```python
from build123d import *

# Parameters (mm, degrees)
F0_W      = 48
F0_H      = 165
F1_DEPTH  = 3
F2_W      = 5.386259
F2_H      = 60
F1_FACE_W = 48
F1_FACE_H = 165
F3_DEPTH  = 3
F4_W      = 15
F4_H      = 17
F5_DEPTH  = 3
F6_R      = 7
F8_DEPTH  = 61.790481
F10_D     = 3
F15_D     = 3
F17_D     = 3
F19_D     = 3
F21_D     = 3


with BuildPart() as f1:
    # F0 (on Top) → F1 (new body)
    with BuildSketch(Plane.XY):
        with Locations((24, 82.5)):
            Rectangle(F0_W, F0_H)
    extrude(amount=F1_DEPTH)

    # F2 (on face) + F1_face (on face) → F3 (join)
    with BuildSketch(Plane.XY.offset(3)):
        with Locations((50.693129, 30)):
            Rectangle(F2_W, F2_H)
    with BuildSketch(Plane(origin=(24, 82.5, 3), x_dir=(1, 0, 0), z_dir=(0, 0, 1))):
        Rectangle(F1_FACE_W, F1_FACE_H)
    extrude(amount=-F3_DEPTH)

    # F4 (on face) → F5 (join)
    with BuildSketch(Plane.XY.offset(3)):
        with Locations((7.5, 173.5)):
            Rectangle(F4_W, F4_H)
    extrude(amount=-F5_DEPTH)

    # F6
    f6_edges = [f1.edges().sort_by_distance(p)[0] for p in [
        (15, 182, 1.5),
    ]]
    fillet(f6_edges, radius=F6_R)

    # F7 (on face) → F8 (cut)
    with BuildSketch(Plane.XY.offset(3)):
        with BuildLine():
            ThreePointArc((52.321299, 55), (49.821299, 57.5), (47.321299, 55))
            Line((47.321299, 55), (47.321299, 5))
            ThreePointArc((47.321299, 5), (49.821299, 2.5), (52.321299, 5))
            Line((52.321299, 5), (52.321299, 55))
        make_face()
    extrude(amount=-F8_DEPTH, mode=Mode.SUBTRACT)

    # F10 (through all)
    with Locations(Plane.XY.offset(3)):
        with Locations((29.321299, 15), (29.321299, 47)):
            Hole(F10_D / 2)

    # F13: F1 across plane


with BuildPart() as f1_1:
    add(f1.part)
    add(f1.part.mirror(Plane.YZ))

    # F15 (through all)
    with Locations(Plane.XY.offset(3)):
        with Locations((6.873526, 174), (-7.126474, 174)):
            Hole(F15_D / 2)

    # F17 (through all)
    with Locations(Plane.XY.offset(3)):
        with Locations((21.825111, 157)):
            Hole(F17_D / 2)

    # F19 (through all)
    with Locations(Plane.XY.offset(3)):
        with Locations((-27.468093, 73), (-27.468093, 158)):
            Hole(F19_D / 2)

    # F21 (through all)
    with Locations(Plane.XY.offset(3)):
        with Locations((39, 74.208118)):
            Hole(F21_D / 2)


solid = f1_1.part
```
Geometry check sheet. Reference: the model listing, model coordinates, mm. Round coordinates to 2 decimals unless told otherwise and drop trailing zeros. Loops run counter-clockwise (first coordinate to the right, second up) from the corner with the lowest first, then second, coordinate; pieces in that order, holes last. Notation, with made-up numbers: (70.25, 68) - (101.25, 68) arc R11 cw to (101.25, 73) - close; hole circle Ø7 at (-21.75, 78.25). An arc over 180 degrees is marked (long way). Write item = value, one per line. Start each with the question number.
1. Thickness scan on line 1 (X direction, y = 8, z = 2.55); line 2 (X direction, y = 73, z = 1.15); line 3 (Y direction, x = 22, z = 2.5). Record the ranges inside material, lowest first.
2. Section check B-B on x = -43.5. Enter the section's corners in (y, z), then the cut area to 3 significant figures.
3. Depth check by flat-ended pin: pin 1 (1 mm diameter, centred on x = 12, z = 1.5, fed in from +Y); pin 2 (2.5 mm diameter, centred on x = 39, y = 74.21, fed in from +Z); pin 3 (0.9 mm diameter, centred on y = 114, z = 1.5, fed in from -X); pin 4 (1.5 mm diameter, centred on x = 49.5, z = 1.5, fed in from +Y). Enter the tip coordinate at first touch or a pass-through.
4. Section check A-A on z = 0.6. Give the number of separate pieces and of enclosed holes in the cut face, then the cut area to 3 significant figures.
5. Section check C-C on y = 98.5. Enter the section's corners in (x, z), then the cut area to 3 significant figures.
Working result:
q1.line_1 = -53.39 to -52.32, -47.32 to 47.32, 52.32 to 53.39
q1.line_2 = -48 to -28.97, -25.97 to 38.11, 39.89 to 48
q1.line_3 = 0 to 155.51, 158.49 to 165
q2.outline = (0, 0) - (165, 0) - (165, 3) - (0, 3) - close
q2.area = 495 mm^2
q3.pin_1 = 181.06
q3.pin_2 = through
q3.pin_3 = -48
q3.pin_4 = 60
q4.separate_pieces = 1
q4.enclosed_holes = 12
q4.area = 16,400 mm^2
q5.outline = (-48, 0) - (48, 0) - (48, 3) - (-48, 3) - close
q5.area = 288 mm^2
